The model under review builds one solid part; all positions refer to its coordinate system, in mm. Face numbers are marked on the shaded views. A direction names the side the tool comes from. Give positions to 0.01 mm unless a question says otherwise; leave off trailing zeros. Loops run counter-clockwise (first coordinate to the right, second up) from the corner with the lowest first, then second, coordinate; pieces in that order, holes last. Notation, with made-up numbers: (34, 10.25) - (78, 10.25) arc R23 cw to (78, 36.25) - close; hole circle Ø3 at (-1, 73.25). An arc over 180 degrees is marked (long way). Return JSON: item names as keys, results as strings. Group by question number.
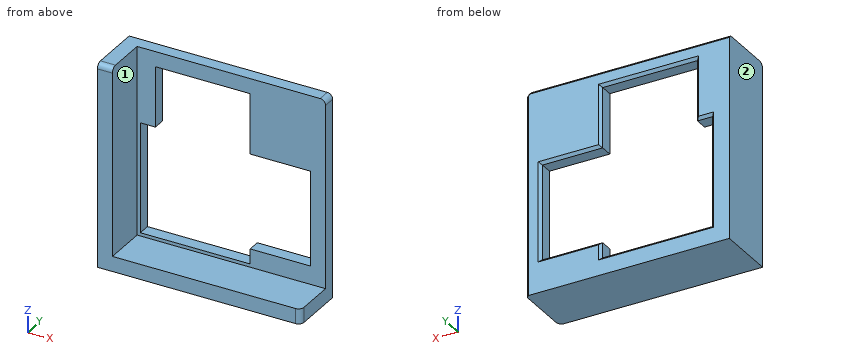
```python
from build123d import *

# Parameters (mm, degrees)
F0_W        = 7
F0_H        = 7
F0_W_2      = 35
F0_H_2      = 52.5
F0_H_3      = 35
F1_DEPTH    = 20
F0_W_3      = 51
F0_H_4      = 1.5
F2_DEPTH    = 7
F3_T1_DEPTH = 19.49950001
F3_T3_DEPTH = 19.49950001
F3_T5_DEPTH = 19.49950001
F4_SIZE     = 1.25


# Not quite as in the source:
# - a fillet or chamfer that OpenCascade refuses, or shapes differently, is made with other operations: its cross-section is extruded or revolved along the edge and cut away or added


with BuildPart() as f1:
    # F0 (on Front) → F1 (new body)
    with BuildSketch(Plane.XZ):
        with Locations((-26.1161934872, -30.8009498573)):
            Rectangle(F0_W, F0_H)
        with Locations((47.3838065128, -30.8009498573)):
            Rectangle(F0_W_2, F0_H)
        with Locations((-26.1161934872, -1.0509498573)):
            Rectangle(F0_W, F0_H_2)
        Polygon((-21.1161934872, -27.3009498573), (-22.6161934872, -27.3009498573), (-22.6161934872, -34.3009498573), (29.8838065128, -34.3009498573), (29.8838065128, -27.3009498573), align=None)
        with Locations((-26.1161934872, 42.6990501427)):
            Rectangle(F0_W, F0_H_3)
    extrude(amount=F1_DEPTH)

    # F0 (on Front) + F1_face (on face) → F2 (join)
    with BuildSketch(Plane.XZ):
        Polygon((-22.6161934872, 60.1990501427), (-22.6161934872, 25.1990501427), (-21.1161934872, 25.1990501427), (-14.1161934872, 25.1990501427), (-14.1161934872, 53.1990501427), (29.8838065128, 53.1990501427), (29.8838065128, 60.1990501427), align=None)
        Polygon((-21.1161934872, -27.3009498573), (-22.6161934872, -27.3009498573), (-22.6161934872, -34.3009498573), (29.8838065128, -34.3009498573), (29.8838065128, -27.3009498573), align=None)
        with Locations((-26.1161934872, 42.6990501427)):
            Rectangle(F0_W, F0_H_3)
        with Locations((-26.1161934872, -1.0509498573)):
            Rectangle(F0_W, F0_H_2)
        Polygon((29.8838065128, -18.8009498573), (29.8838065128, -25.8009498573), (29.8838065128, -27.3009498573), (64.8838065128, -27.3009498573), (64.8838065128, 25.1990501427), (57.8838065128, 25.1990501427), (57.8838065128, -18.8009498573), align=None)
        with Locations((-26.1161934872, -30.8009498573)):
            Rectangle(F0_W, F0_H)
        Polygon((64.8838065128, 60.1990501427), (29.8838065128, 60.1990501427), (29.8838065128, 53.1990501427), (29.8838065128, 25.1990501427), (57.8838065128, 25.1990501427), (64.8838065128, 25.1990501427), align=None)
        with Locations((47.3838065128, -30.8009498573)):
            Rectangle(F0_W_2, F0_H)
        Polygon((-21.1161934872, 25.1990501427), (-22.6161934872, 25.1990501427), (-22.6161934872, -27.3009498573), (-21.1161934872, -27.3009498573), (-21.1161934872, -25.8009498573), align=None)
        with Locations((4.3838065128, -26.5509498573)):
            Rectangle(F0_W_3, F0_H_4)
    with BuildSketch(Plane(origin=(-3.3998473333, -20, -8.0846037034), x_dir=(1, 0, 0), z_dir=(0, -1, 0))):
        Polygon((-26.2163461538, -26.2163461538), (68.2836538462, -26.2163461538), (68.2836538462, -19.2163461538), (-19.2163461538, -19.2163461538), (-19.2163461538, 68.2836538462), (-26.2163461538, 68.2836538462), align=None)
    extrude(amount=F2_DEPTH)

    # F3: fillet of radius 2.5 on 3 edges, made by hand

    # F3_s2 → F3_t1 (cut)
    with BuildSketch(Plane.YZ.offset(-35.8659434922)):
        with BuildLine():
            ThreePointArc((-24.5001, 60.1991501427), (-26.267866953, 59.4669170957), (-27.0001, 57.6991501427))
            Line((-27.0001, 57.6991501427), (-27.0501, 57.6991501427))
            ThreePointArc((-27.0501, 57.6991501427), (-27.05, 58.9491001427), (-27.05, 60.1990501427))
            Line((-27.05, 60.1990501427), (-27, 60.2490501427))
            ThreePointArc((-27, 60.2490501427), (-25.75005, 60.2490501427), (-24.5001, 60.2491501427))
            Line((-24.5001, 60.2491501427), (-24.5001, 60.1991501427))
        make_face()
    extrude(amount=F3_T1_DEPTH, mode=Mode.SUBTRACT)

    # F3_s4 → F3_t3 (cut)
    with BuildSketch(Plane.XY.offset(-40.5506998623)):
        with BuildLine():
            ThreePointArc((64.8839065128, -24.5001), (64.1516734658, -26.267866953), (62.3839065128, -27.0001))
            Line((62.3839065128, -27.0001), (62.3839065128, -27.0501))
            ThreePointArc((62.3839065128, -27.0501), (63.6338565128, -27.05), (64.8838065128, -27.05))
            Line((64.8838065128, -27.05), (64.9338065128, -27))
            ThreePointArc((64.9338065128, -27), (64.9338065128, -25.75005), (64.9339065128, -24.5001))
            Line((64.9339065128, -24.5001), (64.8839065128, -24.5001))
        make_face()
    extrude(amount=F3_T3_DEPTH, mode=Mode.SUBTRACT)

    # F3_s6 → F3_t5 (cut)
    with BuildSketch(Plane.XZ.offset(-6.249750005)):
        with BuildLine():
            ThreePointArc((64.8839065128, 57.6991501427), (64.1516734658, 59.4669170957), (62.3839065128, 60.1991501427))
            Line((62.3839065128, 60.1991501427), (62.3839065128, 60.2491501427))
            ThreePointArc((62.3839065128, 60.2491501427), (63.6338565128, 60.2490501427), (64.8838065128, 60.2490501427))
            Line((64.8838065128, 60.2490501427), (64.9338065128, 60.1990501427))
            ThreePointArc((64.9338065128, 60.1990501427), (64.9338065128, 58.9491001427), (64.9339065128, 57.6991501427))
            Line((64.9339065128, 57.6991501427), (64.8839065128, 57.6991501427))
        make_face()
    extrude(amount=F3_T5_DEPTH, mode=Mode.SUBTRACT)

    # F4
    f4_edges = [f1.edges().sort_by_distance(p)[0] for p in [
        (43.883807, 0, 25.19905),
        (57.883807, 0, 3.19905),
        (43.883807, 0, -18.80095),
        (29.883807, 0, -22.30095),
        (4.383807, 0, -25.80095),
        (-21.116193, 0, -0.30095),
        (29.883807, 0, 39.19905),
        (7.883807, 0, 53.19905),
        (-14.116193, 0, 39.19905),
        (-17.616193, 0, 25.19905),
        (64.883807, 0, 11.71028),
        (16.395037, 0, 60.19905),
        (64.151673, 0, 59.466917),
    ]]
    chamfer(f4_edges, length=F4_SIZE)


solid = f1.part
```
1) We need section C-C, the plane z = 38. Write out the cut boundary in (x, y), plus the area to 3 significant figures.
2) For pin 1 Ø16 at (y, z) = (-14.5, 36) entering from +X; pin 2 Ø5 at (x, z) = (37, -17.5) entering from +Y, all flat-tipped, find the tip position at first contact; note any pin that passes through.
3) We need section D-D, the plane y = -13. Write out the cut boundary in (x, z).
4) We need section B-B, the plane x = 37. Write out the cut boundary in (y, z).
5) We need section A-A, the plane y = -3.25. Write out the cut boundary in (x, z), plus the area to 3 significant figures.
6) To check wall thickness, follow line 1 (X direction, y = -1.75, z = -19); line 2 (X direction, y = -4.75, z = 37.5); line 3 (Z direction, x = -6.5, y = -6). State the ranges of each line that lie inside material, in increasing order.
7) Tool access review of the marked faces 1 and 2: name each direction out of +Z, -Z, +X, -X, +Y, -Y from which nothing blocks a thin tool from reaching the whole face with its end or side.
Findings:
{
 "1": {"outline": "(-29.62, -27) - (-22.62, -27) - (-22.62, -7) - (-14.12, -7) - (-14.12, -1.25) - (-15.37, 0) - (-29.62, 0) - close; (29.88, -7) - (64.88, -7) - (64.88, -1.25) - (63.63, 0) - (31.13, 0) - (29.88, -1.25) - close", "area": "491 mm^2"},
 "2": {"pin 1": "stops at x = 64.88", "pin 2": "stops at y = -0.05"},
 "3": {"outline": "(-29.62, -34.3) - (64.88, -34.3) - (64.88, -27.3) - (-22.62, -27.3) - (-22.62, 60.2) - (-29.62, 60.2) - close"},
 "4": {"outline": "(-27, -34.3) - (0, -34.3) - (0, -20.05) - (-1.25, -18.8) - (-7, -18.8) - (-7, -27.3) - (-27, -27.3) - close; (-7, 25.2) - (-1.25, 25.2) - (0, 26.45) - (0, 58.95) - (-1.25, 60.2) - (-7, 60.2) - close"},
 "5": {"outline": "(-29.62, -34.3) - (64.88, -34.3) - (64.88, 57.72) arc R2.5 ccw to (62.41, 60.2) - (-29.62, 60.2) - close; hole (-21.12, -25.8) - (29.88, -25.8) - (29.88, -18.8) - (57.88, -18.8) - (57.88, 25.2) - (29.88, 25.2) - (29.88, 53.2) - (-14.12, 53.2) - (-14.12, 25.2) - (-21.12, 25.2) - close", "area": "3,860 mm^2"},
 "6": {"line 1": "x = -29.62 to -21.12, 29.88 to 64.88", "line 2": "x = -29.62 to -14.12, 29.88 to 64.88", "line 3": "z = -34.3 to -25.8, 53.2 to 60.2"},
 "7": {"face 1": "+Z, +X, -Y", "face 2": "+Z, -Z, -X, +Y, -Y"}
}
